from build123d import *

# Parameters (mm, degrees)
SKETCH_W        = 388
SKETCH_H        = 369
PAD_DEPTH       = 3
SKETCH001_W     = 25
SKETCH001_H     = 26
SKETCH001_H_2   = 25
POCKET_DEPTH    = 1073.914629
SKETCH002_R     = 12
SKETCH002_R_2   = 1.75
POCKET001_DEPTH = 3.001
SKETCH003_R     = 2.25
POCKET002_DEPTH = 3.001
SKETCH004_W     = 30
SKETCH004_H     = 34
POCKET003_DEPTH = 1073.914629
FILLET_R        = 3
SKETCH005_R     = 5.5
POCKET004_DEPTH = 3.001
SKETCH006_R     = 2.25
POCKET005_DEPTH = 1073.914629
FILLET001_R     = 2
SKETCH007_R     = 5.5
POCKET006_DEPTH = 1073.914629


with BuildPart() as part:
    # Sketch → Pad (new body)
    with BuildSketch(Plane.XY):
        with Locations((0, 0.5)):
            Rectangle(SKETCH_W, SKETCH_H)
    extrude(amount=PAD_DEPTH)

    # Sketch001 (on Face6 of Pad) → Pocket (cut, through all)
    with BuildSketch(Plane.XY.offset(3)):
        with Locations((181.5, 172)):
            Rectangle(SKETCH001_W, SKETCH001_H)
        with Locations((181.5, -171.5)):
            Rectangle(SKETCH001_W, SKETCH001_H_2)
    pocket = extrude(amount=-POCKET_DEPTH, mode=Mode.SUBTRACT)

    # Mirrored: Pocket across YZ
    add(pocket.mirror(Plane.YZ), mode=Mode.SUBTRACT)

    # Sketch002 (on Face4 of Mirrored) → Pocket001 (cut, through all)
    with BuildSketch(Plane.XY.offset(3)):
        with Locations((0, 143)):
            Circle(SKETCH002_R)
        with Locations((-15.5, 158.5)):
            Circle(SKETCH002_R_2)
        with Locations((15.5, 158.5)):
            Circle(SKETCH002_R_2)
        with Locations((15.5, 127.5)):
            Circle(SKETCH002_R_2)
        with Locations((-15.5, 127.5)):
            Circle(SKETCH002_R_2)
        with BuildLine():
            Line((-64, 185), (-50, 185))
            Line((-50, 185), (-50, 143))
            ThreePointArc((-64, 143), (-57, 136), (-50, 143))
            Line((-64, 143), (-64, 185))
        make_face()
        with BuildLine():
            Line((50, 185), (64, 185))
            Line((64, 185), (64, 143))
            ThreePointArc((50, 143), (57, 136), (64, 143))
            Line((50, 143), (50, 185))
        make_face()
    extrude(amount=-POCKET001_DEPTH, mode=Mode.SUBTRACT)

    # Sketch003 (on Face4 of Pocket001) → Pocket002 (cut, through all)
    with BuildSketch(Plane.XY.offset(3)):
        with Locations((125, 175)):
            Circle(SKETCH003_R)
        with Locations((185, 115)):
            Circle(SKETCH003_R)
        with Locations((125, -175)):
            Circle(SKETCH003_R)
        with Locations((-125, 175)):
            Circle(SKETCH003_R)
        with Locations((-185, 115)):
            Circle(SKETCH003_R)
        with Locations((-125, -175)):
            Circle(SKETCH003_R)
        with Locations((0, 175)):
            Circle(SKETCH003_R)
        with Locations((-185, -115)):
            Circle(SKETCH003_R)
        with Locations((185, -115)):
            Circle(SKETCH003_R)
    extrude(amount=-POCKET002_DEPTH, mode=Mode.SUBTRACT)

    # Sketch004 (on Face4 of Pocket002) → Pocket003 (cut, through all)
    with BuildSketch(Plane.XY.offset(3)):
        with Locations((-60, 143)):
            Rectangle(SKETCH004_W, SKETCH004_H)
    pocket003 = extrude(amount=-POCKET003_DEPTH, mode=Mode.SUBTRACT)

    # Mirrored001: Pocket003 across YZ
    add(pocket003.mirror(Plane.YZ), mode=Mode.SUBTRACT)

    # Fillet
    fillet_edges = [part.edges().sort_by_distance(p)[0] for p in [
        (-45, 160, 1.5),
        (-45, 126, 1.5),
        (-75, 126, 1.5),
        (-75, 160, 1.5),
        (45, 126, 1.5),
        (75, 126, 1.5),
        (45, 160, 1.5),
        (75, 160, 1.5),
    ]]
    fillet(fillet_edges, radius=FILLET_R)

    # Sketch005 (on Face52 of Fillet) → Pocket004 (cut, through all)
    with BuildSketch(Plane.XY.offset(3)):
        with Locations((-160, 150)):
            Circle(SKETCH005_R)
        with Locations((-160, -150)):
            Circle(SKETCH005_R)
        with Locations((160, 150)):
            Circle(SKETCH005_R)
        with Locations((160, -150)):
            Circle(SKETCH005_R)
    extrude(amount=-POCKET004_DEPTH, mode=Mode.SUBTRACT)

    # Sketch006 (on Face56 of Pocket004) → Pocket005 (cut, through all)
    with BuildSketch(Plane.XY.offset(3)):
        with Locations((70, 51)):
            Circle(SKETCH006_R)
        with Locations((155, 51)):
            Circle(SKETCH006_R)
        with Locations((70, -75)):
            Circle(SKETCH006_R)
        with Locations((155, -75)):
            Circle(SKETCH006_R)
    pocket005 = extrude(amount=-POCKET005_DEPTH, mode=Mode.SUBTRACT)

    # Mirrored002: Pocket005 across YZ
    add(pocket005.mirror(Plane.YZ), mode=Mode.SUBTRACT)

    # Fillet001
    fillet001_edges = [part.edges().sort_by_distance(p)[0] for p in [
        (169, -159, 1.5),
        (-169, -159, 1.5),
        (-169, 159, 1.5),
        (169, 159, 1.5),
    ]]
    fillet(fillet001_edges, radius=FILLET001_R)

    # Sketch007 (on Face1 of Fillet001) → Pocket006 (cut, through all)
    with BuildSketch(Plane(origin=(0, 0, 0), x_dir=(1, 0, 0), z_dir=(0, 0, -1))):
        with Locations((144.5, -158)):
            Circle(SKETCH007_R)
    pocket006 = extrude(amount=-POCKET006_DEPTH, mode=Mode.SUBTRACT)

    # Mirrored003: Pocket006 across YZ
    add(pocket006.mirror(Plane.YZ), mode=Mode.SUBTRACT)


solid = part.part
CAD build for the part. Positions are in the model's coordinates, mm. Coordinates: 2 decimals unless noted, no trailing zeros. Order: outer loops, then holes, each group sorted by start corner. A loop starts at its lowest first (then second) coordinate and runs counter-clockwise, first axis right, second up.
Item 1: Two-plate mould, pull along Y, no slides. Class faces 1 (the face through (-1.56, 154.9, 1.52)), 2 (the face through (-3, 3, 3)): +Y half, -Y half, draft (parallel to the pull), parting line (faces both ways), or undercut.
Check sheet entries:
face 1: undercut
face 2: draft
Item 2: Band-saw the part on A-A on y = -150. List the corners of the cut face in (x, z).
Check sheet entries:
outline: (-194, 0) - (-165.5, 0) - (-165.5, 3) - (-194, 3) - close; (-154.5, 0) - (154.5, 0) - (154.5, 3) - (-154.5, 3) - close; (165.5, 0) - (194, 0) - (194, 3) - (165.5, 3) - close
Item 3: Band-saw the part on B-B on z = 2.2. Give the number of separate pieces and of enclosed holes in the cut face, plus the area to 3 significant figures.
Check sheet entries:
separate pieces: 1
enclosed holes: 28
area: 137,000 mm2
Item 4: Pin check, flat tip, straight feed: pin 1 Ø0.9 at (x, z) = (-186, 1) entering from +Y. Stop position of the tip, or through.
Check sheet entries:
pin 1: stops at y = 159
Item 5: Drill centre lines: L1, parallel to Y at x = -15.5, z = 2.25; L2, parallel to Y at x = -125, z = 1.6; L3, parallel to X at y = 175, z = 1.3. Where is each one in solid material? Low to high.
Check sheet entries:
L1: y = -184 to 125.75, 129.25 to 156.75, 160.25 to 185
L2: y = -184 to -177.25, -172.75 to 172.75, 177.25 to 185
L3: x = -169 to -127.25, -122.75 to -64, -50 to -2.25, 2.25 to 50, 64 to 122.75, 127.25 to 169
